Source: three-view drawing plus pictorial views. Frame: mm from the lowest corner of the part. Round coordinates to 2 decimals unless told otherwise and drop trailing zeros. Loops run counter-clockwise (first coordinate to the right, second up) from the corner with the lowest first, then second, coordinate; pieces in that order, holes last. Notation, with made-up numbers: M 32,17.25 L 48,17.25 A13 cw 48,30.25 Z; hole C 78.5,-9 d3. An arc over 180 degrees is marked long. Write each question's results on one line, items separated by ' | '.
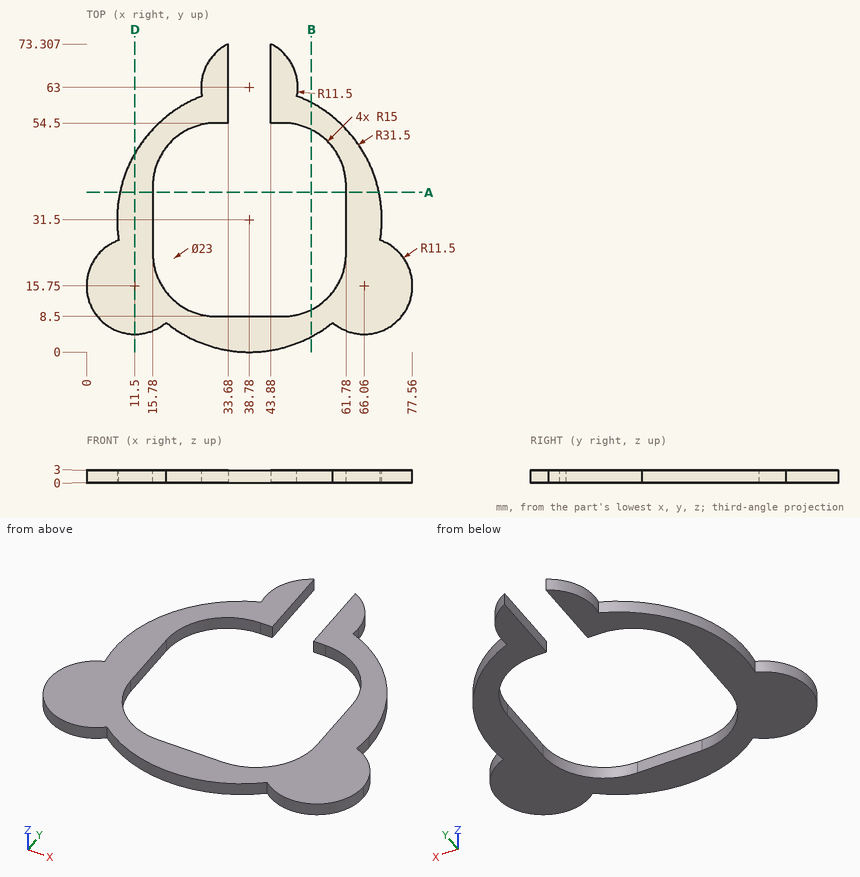
1. Pin query (flat end, axial travel): P1, Ø1.5, axis at y = 30.5, z = 1, coming from the +X side; P2, Ø1.4, axis at x = 45.5, z = 1, coming from the -Y side; P3, Ø0.9, axis at x = 42, z = 2, coming from the +Y side. Return the tip coordinate at first contact, or that it passes through.
Answer key:
P1: stops at x = 70.28 | P2: stops at y = 0.58 | P3: stops at y = 8.5
2. Ray query, probe 1 along X at (y, z) = (31, 0.55) (1 decimal); probe 2 along X at (y, z) = (61, 1.2) (1 decimal); probe 3 along Y at (x, z) = (13, 1.55). Return the intervals inside material, ascending.
Answer key:
probe 1: x = 7.3 to 15.8, 61.8 to 70.3 | probe 2: x = 27.5 to 33.7, 43.9 to 50.1 | probe 3: y = 4.35 to 49.6
3. Section D-D (x = 11.5). Output: boundary loops of the cut face in (y, z), then the cut area to 3 significant figures.
Answer key:
outline: M 4.25,0 L 47.25,0 L 47.25,3 L 4.25,3 Z | area: 129 mm²
4. Section B-B (x = 53.5). Output: boundary loops of the cut face in (y, z).
Answer key:
outline: M 3.65,0 L 10.09,0 L 10.09,3 L 3.65,3 Z; M 52.91,0 L 59.35,0 L 59.35,3 L 52.91,3 Z
5. Section A-A (y = 38). Output: boundary loops of the cut face in (x, z).
Answer key:
outline: M 7.96,0 L 15.78,0 L 15.78,3 L 7.96,3 Z; M 61.78,0 L 69.6,0 L 69.6,3 L 61.78,3 Z
